from build123d import *

# Parameters (mm, degrees)
SKETCH1_W           = 534.67
SKETCH1_H           = 360.934
SKETCH1_W_2         = 528.32
SKETCH1_H_2         = 354.584
BOSS_EXTRUDE1_DEPTH = 203.2
SHELL1_T            = -3.175
SKETCH2_W           = 528.32
SKETCH2_H           = 9.398
CUT_EXTRUDE1_DEPTH  = 493.982347129


with BuildPart() as part:
    # Sketch1 → Boss-Extrude1 (new body)
    # profile 1 of 2: a face of its own
    with BuildSketch(Plane.XY):
        Rectangle(SKETCH1_W, SKETCH1_H)
        Rectangle(SKETCH1_W_2, SKETCH1_H_2, mode=Mode.SUBTRACT)
    # profile 2 of 2: a face of its own
    with BuildSketch(Plane.XY):
        Rectangle(SKETCH1_W_2, SKETCH1_H_2)
    extrude(amount=BOSS_EXTRUDE1_DEPTH)

    # Shell1
    shell1_openings = [part.faces().sort_by_distance(p)[0] for p in [
        (0, 0, 203.2),
    ]]
    offset(amount=SHELL1_T, openings=shell1_openings, kind=Kind.INTERSECTION)

    # Sketch2 → Cut-Extrude1 (cut, through all)
    with BuildSketch(Plane.XZ.offset(180.467)):
        with Locations((0, 7.874)):
            Rectangle(SKETCH2_W, SKETCH2_H)
    extrude(amount=-CUT_EXTRUDE1_DEPTH, mode=Mode.SUBTRACT)


solid = part.part
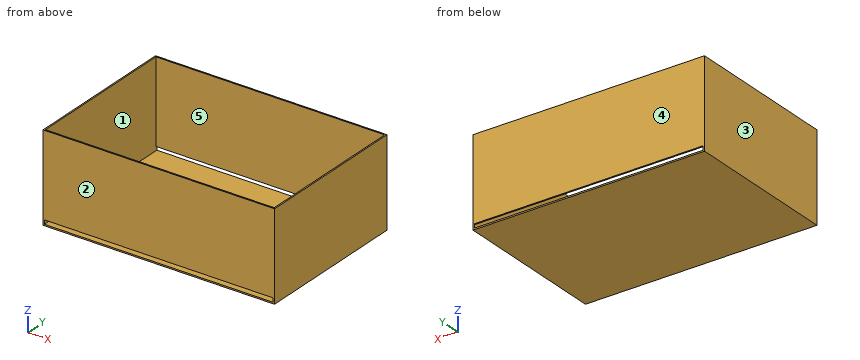
Geometry: final body of the model. Coordinates: model frame, mm. Face numbers are marked on the shaded views. A direction names the side the tool comes from. Coordinates: 2 decimals unless noted, no trailing zeros. Order: outer loops, then holes, each group sorted by start corner. A loop starts at its lowest first (then second) coordinate and runs counter-clockwise, first axis right, second up. Notation, with made-up numbers: (36.25, 20.5) - (76.25, 20.5) arc R22 ccw to (76.25, 26.5) - close; hole circle Ø11 at (39.5, 59). An arc over 180 degrees is marked (long way). Use one line per item in the form item = value.
1) Set-up query: the marked faces 4 and 5. Return all of +Z, -Z, +X, -X, +Y, -Y with unobstructed straight access to the full face (end or side cutting, diameter ignored); none if empty.
Solutions:
face_4 = +Z, -Z, +X, -X, +Y
face_5 = +Z
2) Mould query, pull axis X, two halves, no side actions, for the marked faces 1, 2 and 3. Classes: +X half, -X half, draft (parallel to the pull), parting line (faces both ways), or undercut.
Solutions:
face_1 = undercut
face_2 = draft
face_3 = -X half
3) Ray query, L1, parallel to Y at x = -226, z = 143; L2, parallel to X at y = 133.5, z = 46 (3 decimals); L3, parallel to Z at x = 120, y = -40 (3 decimals). Return the intervals inside material, ascending.
Solutions:
L1 = -180.47 to -177.29, 177.29 to 180.47
L2 = -267.335 to -264.16, 264.16 to 267.335
L3 = 0 to 3.175
4) Section C-C (y = 108.5). Return loops of the section in (x, z) (3 decimals).
Solutions:
outline = (-267.335, 0) - (267.335, 0) - (267.335, 203.2) - (264.16, 203.2) - (264.16, 3.175) - (-264.16, 3.175) - (-264.16, 203.2) - (-267.335, 203.2) - close
5) Section B-B (z = 134). Return loops of the section in (x, y) (3 decimals), then the cut area to 3 significant figures.
Solutions:
outline = (-267.335, -180.467) - (267.335, -180.467) - (267.335, 180.467) - (-267.335, 180.467) - close; hole (-264.16, -177.292) - (264.16, -177.292) - (264.16, 177.292) - (-264.16, 177.292) - close
area = 5,650 mm^2
6) Section A-A (x = 57.5). Return loops of the section in (y, z) (3 decimals), then the cut area to 3 significant figures.
Solutions:
outline = (-180.467, 0) - (180.467, 0) - (180.467, 3.175) - (-180.467, 3.175) - close; (-180.467, 12.573) - (-177.292, 12.573) - (-177.292, 203.2) - (-180.467, 203.2) - close; (177.292, 12.573) - (180.467, 12.573) - (180.467, 203.2) - (177.292, 203.2) - close
area = 2,360 mm^2
